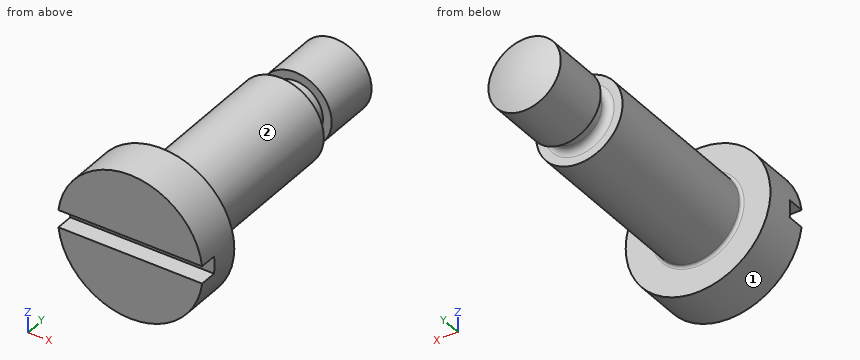
Solid Edge part; units mm, degrees
sketch "Sketch1" plane through (0, 0, 0) normal (0, 0, 1) x (1, 0, 0)
  line L0 (2.985, 12) -> (2.985, 0)
  line L1 (5, 0) -> (2.985, 0)
  line L2 (5, -3.2) -> (5, 0)
  line L3 (0, -3.2) -> (5, -3.2)
  line L4 (0, 0) -> (0, -3.2)
  line L5 (0, 0) -> (0, 12)
  line L6 (0, 12) -> (0, 13.5)
  line L7 (0, 13.5) -> (0, 17.5383)
  line L8 (0, 17.5383) -> (0, 18)
  arc A0 (2.5, 17.5383) -> (0, 18) centre (0, 11) ccw
  line L9 (2.5, 17.5383) -> (2.5, 13.5)
  line L10 (2.5, 13.5) -> (1.9, 13.5)
  line L11 (1.9, 13.5) -> (1.9, 12)
  line L12 (1.9, 12) -> (2.985, 12)
revolve "RevolvedProtrusion1" add sketch "Sketch1" angle 360 about axis through (0, 0, 0) along (0, 1, 0)
fillet "Round1" radius 0.2 1 edges at (0, 0, -2.985)
sketch "Sketch2" plane through (0, -3.2, 0) normal (0, -1, 0) x (1, 0, 0)
  line L0 (-5, 0.6) -> (5, 0.6)
  line L1 (5, 0.6) -> (5, -0.6)
  line L2 (5, -0.6) -> (-5, -0.6)
  line L3 (-5, -0.6) -> (-5, 0.6)
  dimension "D1" = 5
extrude "拉伸除料_1" cut sketch "Sketch2" against normal blind 1.2
fillet "Round2" radius 0.5 1 edges at (0, 12, -1.9)
cosmetic_thread "Thread1"
properties part number "N2611-031B" material "不锈钢 304"
Geometry: final body of the model. Coordinates: model frame, mm. Face numbers are marked on the shaded views. A direction names the side the tool comes from. Round coordinates to 2 decimals unless told otherwise and drop trailing zeros. Order: outer loops, then holes, each group sorted by start corner. A loop starts at its lowest first (then second) coordinate and runs counter-clockwise, first axis right, second up. Notation, with made-up numbers: (9.5, 35) -> (13.5, 35) arc R18 cw to (13.5, 49) -> close; hole circle Ø3 at (18, 7.5). An arc over 180 degrees is marked (long way). Use one line per item in the form item = value.
(1) First-contact query: pin 1 Ø1.5 at (x, y) = (3, 16) entering from +Z; pin 2 Ø1 at (x, z) = (0, 0) entering from -Y; pin 3 Ø1.5 at (x, y) = (3, -1) entering from +Z. Flat tips, straight axial feed; report the tip coordinate or a pass-through.
Results list:
pin_1 = 1.09
pin_2 = -2
pin_3 = 4.47
(2) Access query for the marked faces 1 and 2. Directions: +Z, -Z, +X, -X, +Y, -Y. A direction counts if a zero-diameter tool reaches every point of the face in a straight line with its end or side. Return the directions, or none.
Results list:
face_1 = +Y, -Y
face_2 = +Y
(3) Ray query, probe 1 along Y at (x, z) = (3, -3.5); probe 2 along Y at (x, z) = (-1.25, 2.5); probe 3 along Y at (x, z) = (0, -2). Return the intervals inside material, ascending. Write a range as [from, to].
Results list:
probe_1 = [-3.2, 0]
probe_2 = [-3.2, 12]
probe_3 = [-3.2, 12.2], [13.5, 17.71]
(4) Section C-C on y = 8. Return loops of the section in (x, z) (3 decimals).
Results list:
outline = circle Ø5.97 at (0, 0)
(5) Section A-A on x = 0. Return loops of the section in (y, z) (3 decimals).
Results list:
outline = (-3.2, -5) -> (0, -5) -> (0, -3.185) arc R0.2 cw to (0.2, -2.985) -> (12, -2.985) -> (12, -2.4) arc R0.5 cw to (12.5, -1.9) -> (13.5, -1.9) -> (13.5, -2.5) -> (17.538, -2.5) arc R7 ccw to (17.538, 2.5) -> (13.5, 2.5) -> (13.5, 1.9) -> (12.5, 1.9) arc R0.5 cw to (12, 2.4) -> (12, 2.985) -> (0.2, 2.985) arc R0.2 cw to (0, 3.185) -> (0, 5) -> (-3.2, 5) -> (-3.2, 0.6) -> (-2, 0.6) -> (-2, -0.6) -> (-3.2, -0.6) -> close
(6) Section B-B on z = 0. Return loops of the section in (x, y) (3 decimals).
Results list:
outline = (-5, -2) -> (5, -2) -> (5, 0) -> (3.185, 0) arc R0.2 cw to (2.985, 0.2) -> (2.985, 12) -> (2.4, 12) arc R0.5 cw to (1.9, 12.5) -> (1.9, 13.5) -> (2.5, 13.5) -> (2.5, 17.538) arc R7 ccw to (-2.5, 17.538) -> (-2.5, 13.5) -> (-1.9, 13.5) -> (-1.9, 12.5) arc R0.5 cw to (-2.4, 12) -> (-2.985, 12) -> (-2.985, 0.2) arc R0.2 cw to (-3.185, 0) -> (-5, 0) -> close
(7) Section D-D on z = -4. Return loops of the section in (x, y), and give its area (3 significant figures).
Results list:
outline = (-3, -3.2) -> (3, -3.2) -> (3, 0) -> (-3, 0) -> close
area = 19.2 mm^2
